```python
from build123d import *

# Parameters (mm, degrees)
EXTRUDE_1_DEPTH     = 1
CUT_EXTRUDE_1_DEPTH = 1


with BuildPart() as part:
    # 스케치1 → 보스-돌출1 (new body)
    with BuildSketch(Plane(origin=(0, 0, 0), x_dir=(1, 0, 0), z_dir=(0, 1, 0))):
        with BuildLine():
            Line((-1.4475, -1.73), (1.4475, -1.73))
            Line((1.4475, -1.73), (1.4475, 1.27))
            ThreePointArc((1.4475, 1.27), (0, -8.192062176), (-1.4475, 1.27))
            Line((-1.4475, 1.27), (-1.4475, -1.73))
        make_face()
    extrude(amount=EXTRUDE_1_DEPTH)

    # 스케치2 → 컷-돌출1 (cut)
    with BuildSketch(Plane(origin=(0, 1, 0), x_dir=(1, 0, 0), z_dir=(0, 1, 0))):
        Polygon((-4.080578398, -5.96604295), (-4.305578398, -5.576331518), (-1.707502186, -4.076331518), (-1.482502186, -4.46604295), align=None)
    extrude(amount=-CUT_EXTRUDE_1_DEPTH, mode=Mode.SUBTRACT)


solid = part.part
```
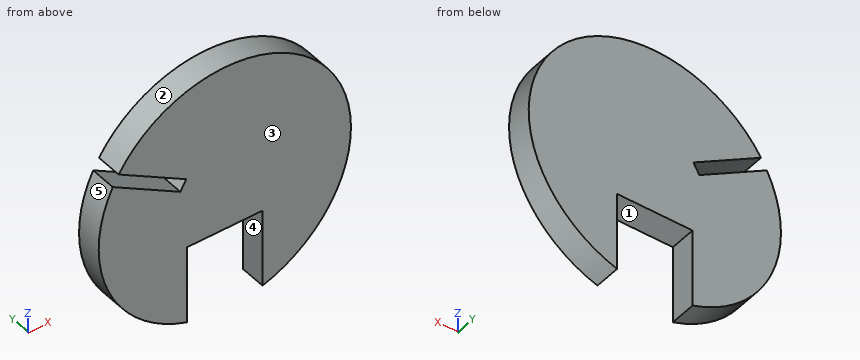
Can you work these out from the model? Positions are in its coordinate system, mm. Face numbers are marked on the shaded views. A direction names the side the tool comes from. Round coordinates to 2 decimals unless told otherwise and drop trailing zeros. Loops run counter-clockwise (first coordinate to the right, second up) from the corner with the lowest first, then second, coordinate; pieces in that order, holes last. Notation, with made-up numbers: (29, 13) -> (49, 13) arc R26 ccw to (49, 29) -> close; hole circle Ø5 at (40, 72.25). An arc over 180 degrees is marked (long way). One line per item, written item: value. Start each with the question number.
1. For the marked faces 1 and 2, which set-ups out of +Z, -Z, +X, -X, +Y, -Y let a thin tool reach every point of the face, with its end or its side?
2. If I drill on probe 1 along X at (y, z) = (0.1, 1); probe 2 along Z at (x, y) = (-3, 0.7); probe 3 along X at (y, z) = (0.95, -1), over which ranges is the centre line in solid material (lowest first)?
3. If we section it at D-D, the plane z = 2.25: Write out the boundary of the cut face in (x, y).
4. If we section it at B-B, the plane y = 0.6: Write out the boundary of the cut face in (x, z).
5. If we mould it in two halves opening along X, with no side actions, what happens to the marked faces 3, 4 and 5? For each: pulls with the +X half, pulls with the -X half, needs draft (parallel to the pull), parting line crosses it, or undercut.
6. If we section it at C-C, the plane x = 0: Write out the boundary of the cut face in (y, z).
7. If we section it at A-A, the plane x = -2.75: Write out the boundary of the cut face in (y, z).
8. For pin 1 (0.5 mm diameter, centred on x = 0, y = 0.5, fed in from -Z), with a flat end and sliding along its axis, tell me the tip position at first contact or that it passes through.
Calculated:
1. face 1: -Z, +Y, -Y
1. face 2: +Y, -Y
2. probe 1: x = -4.23 to -1.45, 1.45 to 4.23
2. probe 2: z = -0.45 to 4.82, 5.34 to 7.15
2. probe 3: x = -2.13 to -1.45, 1.45 to 2.13
3. outline: (-4.72, 0) -> (4.72, 0) -> (4.72, 1) -> (-4.72, 1) -> close
4. outline: (-4.3, 5.57) arc R4.84 ccw to (-1.45, -1.27) -> (-1.45, 1.73) -> (1.45, 1.73) -> (1.45, -1.27) arc R4.84 ccw (long way) to (-4.08, 5.96) -> (-1.48, 4.47) -> (-1.71, 4.08) -> close
5. face 3: needs draft
5. face 4: undercut
5. face 5: pulls with the -X half
6. outline: (0, 1.73) -> (1, 1.73) -> (1, 8.19) -> (0, 8.19) -> close
7. outline: (0, -0.63) -> (1, -0.63) -> (1, 4.68) -> (0, 4.68) -> close; (0, 5.2) -> (1, 5.2) -> (1, 7.34) -> (0, 7.34) -> close
8. pin 1: stops at z = 1.73
